The model under review builds one solid part; all positions refer to its coordinate system, in mm. Face numbers are marked on the shaded views. Coordinates: 2 decimals unless noted, no trailing zeros. Loops run counter-clockwise (first coordinate to the right, second up) from the corner with the lowest first, then second, coordinate; pieces in that order, holes last. Notation, with made-up numbers: M 9,4.5 L 41,4.5 A21 ccw 41,25.5 Z; hole C 52.25,-17.5 d1. An arc over 180 degrees is marked long. One line per item, written item: value.
```python
from build123d import *

# Parameters (mm, degrees)
SKETCH_1_R      = 5
SKETCH_1_R_2    = 1.6
EXTRUDE_1_DEPTH = 3
FILLET_1_R      = 0.5


with BuildPart() as part:
    # ｽｹｯﾁ1 → ﾎﾞｽ - 押し出し1 (new body)
    with BuildSketch(Plane.XY):
        with BuildLine():
            Line((0, 7.5), (15, 7.5))
            Line((15, 7.5), (15, -7.5))
            Line((15, -7.5), (0, -7.5))
            ThreePointArc((0, -7.5), (-7.5, 0), (0, 7.5))
        make_face()
        Circle(SKETCH_1_R, mode=Mode.SUBTRACT)
        with Locations((10, 4.5)):
            Circle(SKETCH_1_R_2, mode=Mode.SUBTRACT)
        with Locations(Location((10, -4.5, 0), (0, 0, 180))):
            Circle(SKETCH_1_R_2, mode=Mode.SUBTRACT)
    extrude(amount=EXTRUDE_1_DEPTH)

    # ﾌｨﾚｯﾄ1
    fillet_1_edges = [part.edges().sort_by_distance(p)[0] for p in [
        (15, 7.5, 1.5),
        (15, -7.5, 1.5),
    ]]
    fillet(fillet_1_edges, radius=FILLET_1_R)


solid = part.part
```
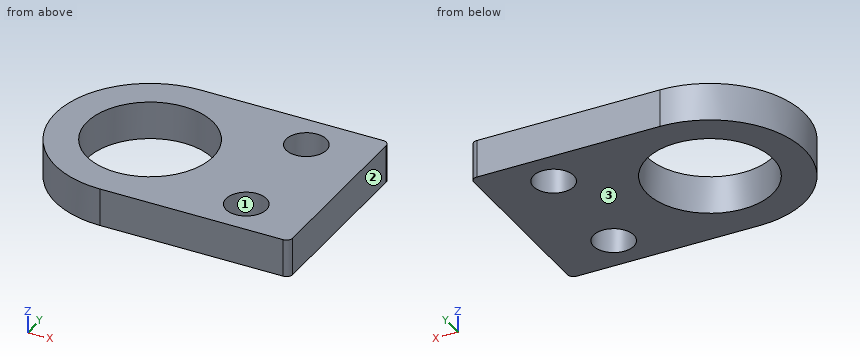
(1) To check wall thickness, follow L1, parallel to Y at x = 10, z = 2.45; L2, parallel to Y at x = 0, z = 2.3; L3, parallel to Y at x = 9.5, z = 2.8. State the ranges of each line that lie inside material, in increasing order. Write a range as [from, to].
Checks:
L1: [-7.5, -6.1], [-2.9, 2.9], [6.1, 7.5]
L2: [-7.5, -5], [5, 7.5]
L3: [-7.5, -6.02], [-2.98, 2.98], [6.02, 7.5]
(2) Draft analysis for pull direction X (two halves, no side actions). For the marked faces 1, 2 and 3, state which applies: pulls with the +X half, pulls with the -X half, needs draft (parallel to the pull), parting line crosses it, or undercut.
Checks:
face 1: undercut
face 2: pulls with the +X half
face 3: needs draft
(3) Add section A-A on y = 0. State the section outline as (x, z) points, then the cut area to 3 significant figures.
Checks:
outline: M -7.5,0 L -5,0 L -5,3 L -7.5,3 Z; M 5,0 L 15,0 L 15,3 L 5,3 Z
area: 37.5 mm^2
(4) Insertion check: pin 1 Ø1.9 at (x, y) = (10, -4.5) entering from -Z. The pin has a flat end and moves straight along its axis. Give the tip position at first contact, or say it passes through.
Checks:
pin 1: through
(5) Add section D-D on x = 2.75. State the section outline as (y, z) points, then the cut area to 3 significant figures.
Checks:
outline: M -7.5,0 L -4.18,0 L -4.18,3 L -7.5,3 Z; M 4.18,0 L 7.5,0 L 7.5,3 L 4.18,3 Z
area: 19.9 mm^2
(6) Add section B-B on z = 1.35. State the section outline as (x, y) points, then the cut area to 3 significant figures.
Checks:
outline: M 0,-7.5 L 14.5,-7.5 A0.5 ccw 15,-7 L 15,7 A0.5 ccw 14.5,7.5 L 0,7.5 A7.5 ccw Z; hole C 0,0 d10; hole C 10,-4.5 d3.2; hole C 10,4.5 d3.2
area: 219 mm^2
(7) Add section C-C on x = 10. State the section outline as (y, z) points, then the cut area to 3 significant figures.
Checks:
outline: M -7.5,0 L -6.1,0 L -6.1,3 L -7.5,3 Z; M -2.9,0 L 2.9,0 L 2.9,3 L -2.9,3 Z; M 6.1,0 L 7.5,0 L 7.5,3 L 6.1,3 Z
area: 25.8 mm^2
